Model file for the job. Use its own axes, mm. Face numbers are marked on the shaded views. A direction names the side the tool comes from. Coordinates: 2 decimals unless noted, no trailing zeros. Order: outer loops, then holes, each group sorted by start corner. A loop starts at its lowest first (then second) coordinate and runs counter-clockwise, first axis right, second up.
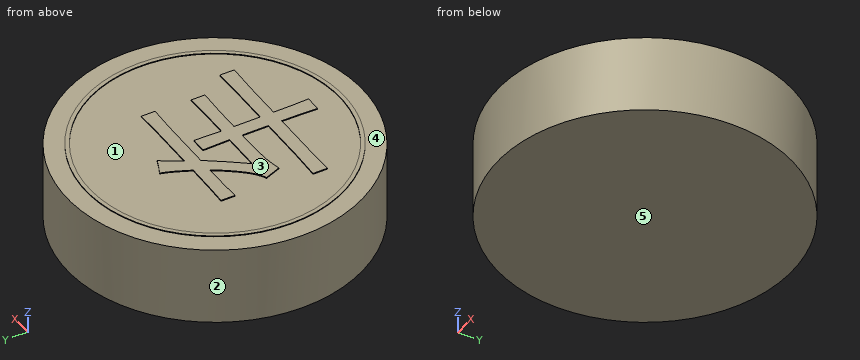
from build123d import *

# Parameters (mm, degrees)
SKETCH_1_R               = 15
DIAMETER30_HEIGHT8_DEPTH = 8
CHARACTER_DEPTH          = 0.1
SKETCH_3_R               = 13.1
SKETCH_3_R_2             = 12.7
INK_RING_DEPTH           = 0.08


with BuildPart() as part:
    # 草图1 → Diameter30_Height8 (new body)
    with BuildSketch(Plane.XY):
        Circle(SKETCH_1_R)
    extrude(amount=-DIAMETER30_HEIGHT8_DEPTH)

    # 草图2 → Character_车 (add)
    with BuildSketch(Plane.XY):
        with BuildLine():
            add(Edge.make_bspline(
                [(-5.842105263, -3.026315789), (-5.898820329, -2.869331425), (-6.006873714, -2.570245254), (-6.168804206, -2.144780878), (-6.320461844, -1.762772614), (-6.42455933, -1.524652502), (-6.473684211, -1.412280702)],
                knots=[0, 0, 0, 0, 1.155372541, 2.201212519, 3.151130129, 4, 4, 4, 4], degree=3))
            add(Edge.make_bspline(
                [(-6.473684211, -1.412280702), (-6.396823444, -1.379800087), (-6.239919961, -1.313494196), (-6.010146568, -1.186156652), (-5.778564765, -1.035723149), (-5.547823353, -0.856912408), (-5.313044861, -0.657208498), (-5.079209262, -0.430138074), (-4.845963085, -0.176973346), (-4.534501394, 0.18732381), (-4.164145867, 0.656391458), (-3.748633816, 1.216101595), (-3.371664409, 1.762234908), (-3.145394749, 2.128474715), (-3.035087719, 2.307017544)],
                knots=[0, 0, 0, 0, 0.584208733, 1.192603045, 1.837360117, 2.517159342, 3.236043131, 3.995784846, 4.79889664, 5.646810753, 7.353001509, 8.984483524, 10.529928116, 12, 12, 12, 12], degree=3))
            add(Edge.make_bspline(
                [(-3.035087719, 2.307017544), (-3.246482619, 2.307526273), (-3.658883418, 2.308518731), (-4.261856974, 2.301476847), (-4.833674599, 2.297370313), (-5.375169247, 2.289752816), (-5.886281193, 2.27816959), (-6.367224064, 2.269967872), (-6.816777836, 2.252736276), (-7.106129451, 2.242011892), (-7.245614035, 2.236842105)],
                knots=[0, 0, 0, 0, 1.204686206, 2.35016811, 3.436405474, 4.463457902, 5.436294372, 6.34989698, 7.204552796, 8, 8, 8, 8], degree=3))
            Line((-7.245614035, 2.236842105), (-7.245614035, 3.640350877))
            add(Edge.make_bspline(
                [(-7.245614035, 3.640350877), (-7.112197092, 3.635099441), (-6.825465539, 3.623813374), (-6.364629063, 3.606862837), (-5.842966328, 3.598841349), (-5.259942843, 3.587169275), (-4.61534822, 3.57975231), (-3.909248078, 3.575626696), (-3.141661522, 3.568632873), (-2.609705057, 3.569648027), (-2.333333333, 3.570175439)],
                knots=[0, 0, 0, 0, 0.652233806, 1.401741091, 2.25255631, 3.200691931, 4.250322975, 5.401478114, 6.649968519, 8, 8, 8, 8], degree=3))
            add(Edge.make_bspline(
                [(-2.333333333, 3.570175439), (-2.265182445, 3.706781651), (-2.13249513, 3.972749008), (-1.948730322, 4.364802108), (-1.781805751, 4.736299128), (-1.633474827, 5.088418502), (-1.500571846, 5.419860952), (-1.385562669, 5.732537711), (-1.288604233, 6.025373857), (-1.235803724, 6.215836544), (-1.210526316, 6.307017544)],
                knots=[0, 0, 0, 0, 1.236548776, 2.407515765, 3.506966959, 4.535340541, 5.502281012, 6.399229081, 7.23365623, 8, 8, 8, 8], degree=3))
            add(Edge.make_bspline(
                [(-1.210526316, 6.307017544), (-1.072464078, 6.238250423), (-0.801072324, 6.103073492), (-0.390506761, 5.92371698), (0.006858558, 5.752049753), (0.273104458, 5.653521307), (0.403508772, 5.605263158)],
                knots=[0, 0, 0, 0, 1.050893361, 2.065762486, 3.052631741, 4, 4, 4, 4], degree=3))
            add(Edge.make_bspline(
                [(0.403508772, 5.605263158), (0.287716291, 5.440743002), (0.057094455, 5.113071117), (-0.262779106, 4.605286149), (-0.575699306, 4.095748706), (-0.765073243, 3.745229449), (-0.859649123, 3.570175439)],
                knots=[0, 0, 0, 0, 1.007065107, 2.005753766, 3.00404673, 4, 4, 4, 4], degree=3))
            Line((-0.859649123, 3.570175439), (3.912280702, 3.570175439))
            add(Edge.make_bspline(
                [(3.912280702, 3.570175439), (3.986792128, 3.569779735), (4.146229603, 3.568933021), (4.399164705, 3.576215116), (4.681635542, 3.580205028), (4.991801347, 3.588183635), (5.330489118, 3.599673551), (5.697948203, 3.608156571), (6.093748619, 3.625727153), (6.367546823, 3.635374682), (6.50877193, 3.640350877)],
                knots=[0, 0, 0, 0, 0.688397439, 1.473013676, 2.337661006, 3.298515698, 4.339608953, 5.468714639, 6.694363069, 8, 8, 8, 8], degree=3))
            Line((6.50877193, 3.640350877), (6.50877193, 2.236842105))
            add(Edge.make_bspline(
                [(6.50877193, 2.236842105), (6.279214943, 2.247975922), (5.82888106, 2.269817709), (5.1668562, 2.289395513), (4.530922728, 2.303382911), (4.115883288, 2.305821342), (3.912280702, 2.307017544)],
                knots=[0, 0, 0, 0, 1.061662981, 2.082719505, 3.05945501, 4, 4, 4, 4], degree=3))
            Line((3.912280702, 2.307017544), (-1.49122807, 2.307017544))
            add(Edge.make_bspline(
                [(-1.49122807, 2.307017544), (-1.56117399, 2.201167925), (-1.710872673, 1.974627926), (-1.95506101, 1.616085811), (-2.235185889, 1.218787258), (-2.555254083, 0.784910796), (-2.903437302, 0.30729052), (-3.289360757, -0.207943656), (-3.711097719, -0.76191269), (-4.005224498, -1.143853854), (-4.157894737, -1.342105263)],
                knots=[0, 0, 0, 0, 0.673545103, 1.441525336, 2.302896076, 3.254132591, 4.303779702, 5.440759354, 6.671593656, 8, 8, 8, 8], degree=3))
            Line((-4.157894737, -1.342105263), (-0.228070175, -1.342105263))
            add(Edge.make_bspline(
                [(-0.228070175, -1.342105263), (-0.231461537, -0.891528138), (-0.238331174, 0.021173694), (-0.278106388, 0.933036802), (-0.298245614, 1.394736842)],
                knots=[0, 0, 0, 0, 0.987347913, 2, 2, 2, 2], degree=3))
            Line((-0.298245614, 1.394736842), (1.245614035, 1.394736842))
            add(Edge.make_bspline(
                [(1.245614035, 1.394736842), (1.234342441, 1.188579897), (1.211003525, 0.761712205), (1.192285381, 0.099612341), (1.178632375, -0.606505386), (1.176525709, -1.091718406), (1.175438596, -1.342105263)],
                knots=[0, 0, 0, 0, 0.904818853, 1.873514066, 2.902659025, 4, 4, 4, 4], degree=3))
            Line((1.175438596, -1.342105263), (3.561403509, -1.342105263))
            add(Edge.make_bspline(
                [(3.561403509, -1.342105263), (4.023251472, -1.338996907), (4.935977079, -1.332854028), (5.847809296, -1.292074512), (6.298245614, -1.271929825)],
                knots=[0, 0, 0, 0, 1.012019295, 2, 2, 2, 2], degree=3))
            Line((6.298245614, -1.271929825), (6.298245614, -2.675438596))
            add(Edge.make_bspline(
                [(6.298245614, -2.675438596), (5.847809296, -2.655293909), (4.935977079, -2.614514393), (4.023251472, -2.608371514), (3.561403509, -2.605263158)],
                knots=[0, 0, 0, 0, 0.987980705, 2, 2, 2, 2], degree=3))
            Line((3.561403509, -2.605263158), (1.175438596, -2.605263158))
            Line((1.175438596, -2.605263158), (1.175438596, -5.271929825))
            Line((1.175438596, -5.271929825), (5.105263158, -5.271929825))
            add(Edge.make_bspline(
                [(5.105263158, -5.271929825), (5.333122844, -5.270715306), (5.801003783, -5.268221447), (6.520106526, -5.254311899), (7.274811493, -5.234595053), (7.789282241, -5.212873368), (8.052631579, -5.201754386)],
                knots=[0, 0, 0, 0, 0.927389459, 1.904276523, 2.92723271, 4, 4, 4, 4], degree=3))
            Line((8.052631579, -5.201754386), (8.052631579, -6.675438596))
            add(Edge.make_bspline(
                [(8.052631579, -6.675438596), (7.789282241, -6.664319614), (7.274811493, -6.64259793), (6.520106526, -6.622881083), (5.801003783, -6.608971535), (5.333122844, -6.606477676), (5.105263158, -6.605263158)],
                knots=[0, 0, 0, 0, 1.07276729, 2.095723477, 3.072610541, 4, 4, 4, 4], degree=3))
            Line((5.105263158, -6.605263158), (1.175438596, -6.605263158))
            add(Edge.make_bspline(
                [(1.175438596, -6.605263158), (1.17492319, -6.788068469), (1.173921664, -7.143291287), (1.180988322, -7.662224869), (1.185055025, -8.151741366), (1.192680502, -8.613534144), (1.204276819, -9.04666503), (1.212388046, -9.451393023), (1.229724118, -9.827285169), (1.240445713, -10.06811771), (1.245614035, -10.184210526)],
                knots=[0, 0, 0, 0, 1.225493371, 2.381348807, 3.479127077, 4.507295234, 5.477513674, 6.383863443, 7.220944797, 8, 8, 8, 8], degree=3))
            Line((1.245614035, -10.184210526), (-0.298245614, -10.184210526))
            add(Edge.make_bspline(
                [(-0.298245614, -10.184210526), (-0.293088467, -10.062919018), (-0.28244323, -9.812552555), (-0.26517016, -9.425394066), (-0.256955584, -9.014609066), (-0.245308677, -8.579745809), (-0.237743343, -8.120551737), (-0.233625145, -7.637100266), (-0.226569426, -7.129429714), (-0.227561666, -6.782870303), (-0.228070175, -6.605263158)],
                knots=[0, 0, 0, 0, 0.813876, 1.679979569, 2.597948426, 3.568174058, 4.596349836, 5.676713029, 6.809345956, 8, 8, 8, 8], degree=3))
            Line((-0.228070175, -6.605263158), (-5.070175439, -6.605263158))
            add(Edge.make_bspline(
                [(-5.070175439, -6.605263158), (-5.324893201, -6.606388994), (-5.827429759, -6.608610173), (-6.573394245, -6.622429105), (-7.301292576, -6.641441143), (-7.781058, -6.664213602), (-8.01754386, -6.675438596)],
                knots=[0, 0, 0, 0, 1.036669794, 2.04526165, 3.036470834, 4, 4, 4, 4], degree=3))
            Line((-8.01754386, -6.675438596), (-8.01754386, -5.201754386))
            add(Edge.make_bspline(
                [(-8.01754386, -5.201754386), (-7.781058, -5.212979381), (-7.301292576, -5.235751839), (-6.573394245, -5.254763877), (-5.827429759, -5.268582809), (-5.324893201, -5.270803988), (-5.070175439, -5.271929825)],
                knots=[0, 0, 0, 0, 0.963529166, 1.95473835, 2.963330206, 4, 4, 4, 4], degree=3))
            Line((-5.070175439, -5.271929825), (-0.228070175, -5.271929825))
            Line((-0.228070175, -5.271929825), (-0.228070175, -2.605263158))
            add(Edge.make_bspline(
                [(-0.228070175, -2.605263158), (-0.430801667, -2.604732204), (-0.819811605, -2.603713387), (-1.378600845, -2.610674903), (-1.888907343, -2.614839935), (-2.351576194, -2.622216615), (-2.76650508, -2.633903903), (-3.133156573, -2.641670696), (-3.450969213, -2.659258343), (-3.813777921, -2.677582124), (-4.243119388, -2.723022723), (-4.761241386, -2.794248367), (-5.296964879, -2.896480162), (-5.65789017, -2.982441435), (-5.842105263, -3.026315789)],
                knots=[0, 0, 0, 0, 1.292465027, 2.480037691, 3.562671594, 4.545968376, 5.429981271, 6.209087619, 6.883751335, 7.459135407, 8.52479941, 9.634773871, 10.792796285, 12, 12, 12, 12], degree=3))
        make_face()
    extrude(amount=CHARACTER_DEPTH)

    # 草图3 → Ink_ring (add)
    with BuildSketch(Plane.XY):
        with Locations(Location((0, 0, 0), (0, 0, 180))):
            Circle(SKETCH_3_R)
        with Locations(Location((0, 0, 0), (0, 0, 180))):
            Circle(SKETCH_3_R_2, mode=Mode.SUBTRACT)
    extrude(amount=INK_RING_DEPTH)


solid = part.part
Q1. Cut at B-B, the plane x = -12.25. List the corners of the cut face in (y, z).
Established:
outline: (-8.66, -8) - (8.66, -8) - (8.66, 0) - (4.64, 0) - (4.64, 0.08) - (3.35, 0.08) - (3.35, 0) - (-3.35, 0) - (-3.35, 0.08) - (-4.64, 0.08) - (-4.64, 0) - (-8.66, 0) - close
Q2. Mould opens along Y. For the marked faces 1, 2 and 3 say: pulls with the +Y half, pulls with the -Y half, needs draft (parallel to the pull), parting line crosses it, or undercut.
Established:
face 1: undercut
face 2: parting line crosses it
face 3: needs draft
Q3. Cut at A-A, the plane y = 10. List the corners of the cut face in (x, z), plus the area to 3 significant figures.
Established:
outline: (-11.18, -8) - (11.18, -8) - (11.18, 0) - (8.46, 0) - (8.46, 0.08) - (7.83, 0.08) - (7.83, 0) - (-7.83, 0) - (-7.83, 0.08) - (-8.46, 0.08) - (-8.46, 0) - (-11.18, 0) - close
area: 179 mm2
Q4. Which spindle directions (+Z, -Z, +X, -X, +Y, -Y) get a long thin tool onto all of the face, cutting with end or side? Do the marked faces 4 and 5. Say none if no direction does.
Established:
face 4: +Z
face 5: -Z, +X, -X, +Y, -Y
Q5. Cut at C-C, the plane z = -1. List the corners of the cut face in (x, y), plus the area to 3 significant figures.
Established:
outline: circle Ø30 at (0, 0)
area: 707 mm2
Q6. Drop flat-ended pins along their axis: P1, Ø3, axis at y = -3, z = -7, coming from the -X side; P2, Ø4, axis at x = 3.5, z = -3.5, coming from the -Y side; P3, Ø2, axis at y = -6, z = -1, coming from the -X side. Give the stop position or say it passes through.
Established:
P1: stops at x = -14.92
P2: stops at y = -14.92
P3: stops at x = -14.14
Q7. Probe line 1 (Z direction, x = -1, y = 8.75); line 2 (Z direction, x = 3.5, y = -12.5); line 3 (X direction, y = 2.75, z = -4.25). List the from-to ranges inside material, lowest first.
Established:
line 1: z = -8 to 0
line 2: z = -8 to 0.08
line 3: x = -14.75 to 14.75
